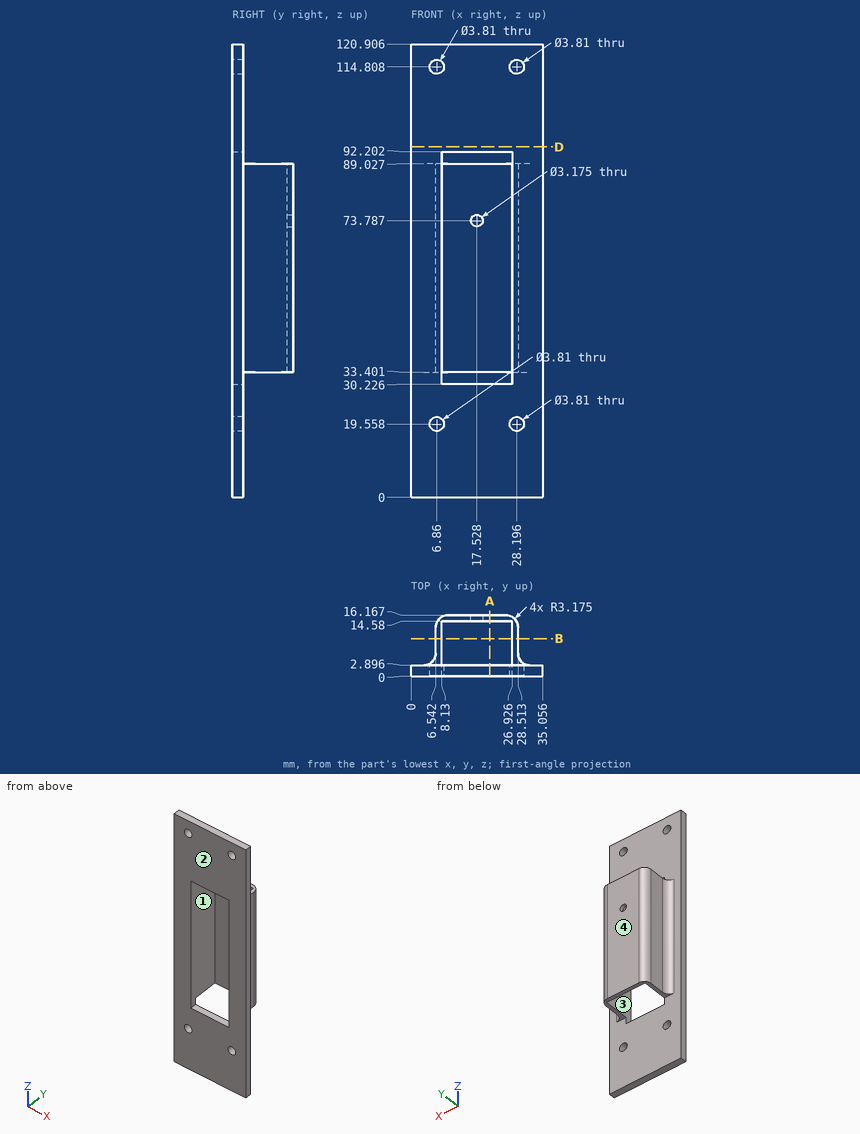
Verification items for this drawing (mm, ordinates from the low corner). A direction names the side the tool comes from. Coordinates: 2 decimals unless noted, no trailing zeros. Loops run counter-clockwise (first coordinate to the right, second up) from the corner with the lowest first, then second, coordinate; pieces in that order, holes last.
Item 1: Go/stop test with flat-tipped pins: pin 1 Ø4 at (x, y) = (11.5, 8.5) entering from -Z (3 decimals); pin 2 Ø2 at (y, z) = (10.5, 62) entering from -X; pin 3 Ø1 at (x, y) = (28, 7) entering from -Z; pin 4 Ø5.5 at (x, z) = (17.5, 55) entering from -Y. Record where each tip stops, or that it passes through.
Item 2: Release check for a two-part mould opening along X. For the marked faces 3 and 4 record: released by +X, released by -X, zero draft, split by the parting line, or undercut.
Item 3: Sectioned sample at B-B, the plane y = 10. Record the boundary of the cut face in (x, z) (1 decimal).
Item 4: Sectioned sample at A-A, the plane x = 21. Record the boundary of the cut face in (y, z) (1 decimal).
Item 5: Thickness scan on line 1 (Z direction, x = 6.86, y = 1.5) (1 decimal); line 2 (X direction, y = 13, z = 72) (1 decimal); line 3 (X direction, y = 1, z = 76) (1 decimal). Record the ranges inside material, lowest first.
Item 6: Sectioned sample at D-D, the plane z = 93.5. Record the boundary of the cut face in (x, y) (1 decimal).
Item 7: Access from +Z, -Z, +X, -X, +Y, -Y to the whole of each face (thin tool, end or side, straight path). Record for the marked faces 1 and 2.
Check result:
1. pin 1: passes through
1. pin 2: stops at x = 6.54
1. pin 3: stops at z = 33.4
1. pin 4: stops at y = 14.58
2. face 3: undercut
2. face 4: zero draft
3. outline: (6.5, 33.4) - (8.1, 33.4) - (8.1, 89) - (6.5, 89) - close; (26.9, 33.4) - (28.5, 33.4) - (28.5, 89) - (26.9, 89) - close
4. outline: (0, 0) - (2.9, 0) - (2.9, 30.2) - (0, 30.2) - close; (0, 92.2) - (2.9, 92.2) - (2.9, 120.9) - (0, 120.9) - close; (14.6, 33.4) - (16.2, 33.4) - (16.2, 89) - (14.6, 89) - close
5. line 1: z = 0 to 17.7, 21.5 to 112.9, 116.7 to 120.9
5. line 2: x = 6.5 to 8.1, 26.9 to 28.5
5. line 3: x = 0 to 8.1, 26.9 to 35.1
6. outline: (0, 0) - (35.1, 0) - (35.1, 2.9) - (0, 2.9) - close
7. face 1: -Y
7. face 2: +Z, -Z, +X, -X, -Y
